```python
from build123d import *

# Parameters (mm, degrees)
F2_R = 0.99999
F3_R = 0.99999


# Not quite as in the source:
# - a fillet or chamfer is up to 0.001 mm smaller than in the source, because OpenCascade refuses the exact size


with BuildPart() as f1:
    # F0 (on Top) → F1 (revolve)
    with BuildSketch(Plane.XY):
        Polygon((25, 7), (25, 0), (28, 0), (28, 2), (26, 2), (26, 7), align=None)
    revolve(axis=Axis((0, 6.8999978745, 0), (0, 1, 0)))

    # F2 (radius 1 in the source; OpenCascade refuses exactly that, so slightly less here)
    f2_edges = [f1.edges().sort_by_distance(p)[0] for p in [
        (-26, 2, 0),
        (-28, 2, 0),
    ]]
    fillet(f2_edges, radius=F2_R)

    # F3 (radius 1 in the source; OpenCascade refuses exactly that, so slightly less here)
    f3_edges = [f1.edges().sort_by_distance(p)[0] for p in [
        (-26, 7, 0),
    ]]
    fillet(f3_edges, radius=F3_R)


solid = f1.part
```
Can you work these out from the model? Positions are in its coordinate system, mm. Coordinates: 2 decimals unless noted, no trailing zeros. Order: outer loops, then holes, each group sorted by start corner. A loop starts at its lowest first (then second) coordinate and runs counter-clockwise, first axis right, second up.
1. Thinking about a two-plate mould opening in Z: for faces 1 (the face through (-20.633, 4.521, 15.821)), 2 (the face through (11, 0, -23)), 3 (the face through (23.846, 3.451, -7.509)), which applies, +Z half, -Z half, draft (parallel to the pull), parting line (faces both ways), or undercut?
2. I need wall thicknesses on line 1 (X direction, y = 3.5, z = 0); line 2 (X direction, y = 1, z = 21); line 3 (Z direction, x = -17, y = 4.5). Which ranges of each line are inside material? Lowest first, please.
3. I'm going to push flat-ended pins straight in: pin 1 (1.5 mm diameter, centred on y = 5.5, z = 5, fed in from +X); pin 2 (1 mm diameter, centred on y = 1, z = -11, fed in from -X); pin 3 (1 mm diameter, centred on x = -20.5, y = 3.5, fed in from -Z). Where does each tip first touch, or does it pass through?
4. If we section it at C-C (y = 4): Please give me the cut outline in (x, z), then the cut area to 3 significant figures.
Entries:
1. face 1: parting line
1. face 2: draft
1. face 3: undercut
2. line 1: x = -26 to -25, 25 to 26
2. line 2: x = -18.52 to -13.56, 13.56 to 18.52
2. line 3: z = -19.67 to -18.33, 18.33 to 19.67
3. pin 1: stops at x = 25.65
3. pin 2: stops at x = -25.96
3. pin 3: stops at z = -16.61
4. outline: circle Ø52 at (0, 0); hole circle Ø50 at (0, 0)
4. area: 160 mm2
